Could you check a few things on this model? Use its own coordinates, in mm. A direction names the side the tool comes from. Round coordinates to 2 decimals unless told otherwise and drop trailing zeros. Loops run counter-clockwise (first coordinate to the right, second up) from the corner with the lowest first, then second, coordinate; pieces in that order, holes last. Notation, with made-up numbers: (21, 87.25) -> (69, 87.25) arc R29 ccw to (69, 120.25) -> close; hole circle Ø4 at (72, 59). An arc over 180 degrees is marked (long way). One line per item, written item: value.
from build123d import *

# Parameters (mm, degrees)
EXTRUDE_1_DEPTH     = 40
SKETCH_2_W          = 75
SKETCH_2_H          = 12
CUT_EXTRUDE_1_DEPTH = 73.284161474


with BuildPart() as part:
    # Эскиз1 → Бобышка-Вытянуть1 (new body)
    with BuildSketch(Plane.XY):
        with BuildLine():
            Line((45, -40), (45, 40))
            Line((45, 40), (-45, 40))
            Line((-45, 40), (-45, 21.5))
            ThreePointArc((-45, 21.5), (-23.5, 0), (-45, -21.5))
            Line((-45, -21.5), (-45, -40))
            Line((-45, -40), (45, -40))
        make_face()
        with BuildLine():
            ThreePointArc((-4.5, -23), (-13, -14.5), (-4.5, -6))
            Line((-4.5, -6), (26.5, -6))
            ThreePointArc((26.5, -6), (35, -14.5), (26.5, -23))
            Line((26.5, -23), (-4.5, -23))
        make_face(mode=Mode.SUBTRACT)
        with BuildLine():
            Line((26.5, 6), (-4.5, 6))
            ThreePointArc((-4.5, 6), (-13, 14.5), (-4.5, 23))
            Line((-4.5, 23), (26.5, 23))
            ThreePointArc((26.5, 23), (35, 14.5), (26.5, 6))
        make_face(mode=Mode.SUBTRACT)
    extrude(amount=EXTRUDE_1_DEPTH)

    # Эскиз2 → Вырез-Вытянуть1 (cut, through all)
    with BuildSketch(Plane.XY.offset(40)):
        with Locations((7.5, 34)):
            Rectangle(SKETCH_2_W, SKETCH_2_H)
    cut_extrude_1 = extrude(amount=-CUT_EXTRUDE_1_DEPTH, mode=Mode.SUBTRACT)

    # Зеркальное отражение1: Вырез-Вытянуть1 across plane
    add(cut_extrude_1.mirror(Plane.ZX), mode=Mode.SUBTRACT)


solid = part.part
(1) For faces 5 (the face through (7, -28, 20)), 6 (the face through (7, 28, 20)), 7 (the face through (11, 23, 20)), 8 (the face through (-38, -40, 20)), which set-ups out of +Z, -Z, +X, -X, +Y, -Y let a thin tool reach every point of the face, with its end or its side?
Recorded:
face 5: +Z, -Z, +X, -Y
face 6: +Z, -Z, +X, +Y
face 7: +Z, -Z
face 8: +Z, -Z, +X, -X, -Y
(2) If we section it at C-C, the plane y = -14.5: Please give me the cut outline in (x, z).
Recorded:
outline: (-29.13, 0) -> (-13, 0) -> (-13, 40) -> (-29.13, 40) -> close; (35, 0) -> (45, 0) -> (45, 40) -> (35, 40) -> close
(3) If we section it at B-B, the plane z = 23.5: Please give me the cut outline in (x, y), then the cut area to 3 significant figures.
Recorded:
outline: (-45, -40) -> (-30, -40) -> (-30, -28) -> (45, -28) -> (45, 28) -> (-30, 28) -> (-30, 40) -> (-45, 40) -> (-45, 21.5) arc R21.5 cw to (-45, -21.5) -> close; hole (-4.5, -23) -> (26.5, -23) arc R8.5 ccw to (26.5, -6) -> (-4.5, -6) arc R8.5 ccw to start; hole (-4.5, 6) -> (26.5, 6) arc R8.5 ccw to (26.5, 23) -> (-4.5, 23) arc R8.5 ccw to start
area: 3,170 mm²
(4) If we section it at A-A, the plane x = 30.5: Please give me the cut outline in (y, z), then the cut area to 3 significant figures.
Recorded:
outline: (-28, 0) -> (-22, 0) -> (-22, 40) -> (-28, 40) -> close; (-7, 0) -> (7, 0) -> (7, 40) -> (-7, 40) -> close; (22, 0) -> (28, 0) -> (28, 40) -> (22, 40) -> close
area: 1,040 mm²
(5) I'm going to push flat-ended pins straight in: pin 1 Ø5 at (y, z) = (-15.5, 6) entering from -X; pin 2 Ø1.5 at (x, z) = (-28.5, 24.5) entering from -Y; pin 3 Ø6 at (y, z) = (-32, 24) entering from +X. Where does each tip first touch, or does it pass through?
Recorded:
pin 1: x = -33.24
pin 2: y = -28
pin 3: x = -30
(6) If we section it at D-D, the plane x = -35: Please give me the cut outline in (y, z), then the cut area to 3 significant figures.
Recorded:
outline: (-40, 0) -> (-19.03, 0) -> (-19.03, 40) -> (-40, 40) -> close; (19.03, 0) -> (40, 0) -> (40, 40) -> (19.03, 40) -> close
area: 1,680 mm²
(7) If I drill on L1, parallel to Y at x = 26, z = 5; L2, parallel to Y at x = -7.5, z = 18; L3, parallel to X at y = 35, z = 29.5, over which ranges is the centre line in solid material (lowest first)?
Recorded:
L1: -28 to -23, -6 to 6, 23 to 28
L2: -28 to -22.45, -6.55 to 6.55, 22.45 to 28
L3: -45 to -30
(8) Thinking about a two-plate mould opening in X: for faces 1 (the face through (11, 6, 20)), 2 (the face through (45, 0, 20)), 3 (the face through (-23.505, 0.473, 19.72)), 4 (the face through (-1, 1, 0)), which applies, released by +X, released by -X, zero draft, split by the parting line, or undercut?
Recorded:
face 1: undercut
face 2: released by +X
face 3: released by -X
face 4: zero draft
